Check sheet for the modelled part. Datum: model origin and axes. Units: mm. A direction names the side the tool comes from. Round coordinates to 2 decimals unless told otherwise and drop trailing zeros. Loops run counter-clockwise (first coordinate to the right, second up) from the corner with the lowest first, then second, coordinate; pieces in that order, holes last. Notation, with made-up numbers: (-28, 63.5) - (-13, 63.5) arc R11 cw to (-13, 72.5) - close; hole circle Ø4 at (60, 62). An arc over 180 degrees is marked (long way). Put each result on its own line as item: value.
```python
from build123d import *

# Parameters (mm, degrees)
SKETCH_R        = 31.9
SKETCH_R_2      = 6
PAD_DEPTH       = 2
SKETCH001_R     = 31.9
SKETCH001_R_2   = 30
PAD001_DEPTH    = 2
PAD002_DEPTH    = 2
CHAMFER_SIZE    = 1.9
CHAMFER001_SIZE = 0.3


with BuildPart() as part:
    # Sketch → Pad (new body)
    with BuildSketch(Plane.XY):
        Circle(SKETCH_R)
        with Locations((9.999037, 20.71278)):
            Circle(SKETCH_R_2, mode=Mode.SUBTRACT)
        with Locations((22.937312, 1.69697)):
            Circle(SKETCH_R_2, mode=Mode.SUBTRACT)
        with Locations((12.938275, -19.01581)):
            Circle(SKETCH_R_2, mode=Mode.SUBTRACT)
        with Locations((-9.999037, -20.71278)):
            Circle(SKETCH_R_2, mode=Mode.SUBTRACT)
        with Locations((-22.937312, -1.69697)):
            Circle(SKETCH_R_2, mode=Mode.SUBTRACT)
        with Locations((-12.938275, 19.01581)):
            Circle(SKETCH_R_2, mode=Mode.SUBTRACT)
        Polygon((0, 16.858628), (-14.6, 8.429314), (-14.6, -8.429314), (0, -16.858628), (14.6, -8.429314), (14.6, 8.429314), align=None, mode=Mode.SUBTRACT)
    extrude(amount=PAD_DEPTH)

    # Sketch001 (on Face15 of Pad) → Pad001 (join)
    with BuildSketch(Plane.XY.offset(2)):
        Circle(SKETCH001_R)
        Circle(SKETCH001_R_2, mode=Mode.SUBTRACT)
    extrude(amount=PAD001_DEPTH)

    # Sketch002 (on Face17 of Pad001) → Pad002 (join)
    with BuildSketch(Plane.XY.offset(2)):
        Polygon((0, 19.052559), (-16.5, 9.526279), (-16.5, -9.526279), (0, -19.052559), (16.5, -9.526279), (16.5, 9.526279), align=None)
        Polygon((0, 16.858628), (-14.6, 8.429314), (-14.6, -8.429314), (0, -16.858628), (14.6, -8.429314), (14.6, 8.429314), align=None, mode=Mode.SUBTRACT)
    extrude(amount=PAD002_DEPTH)

    # Chamfer
    chamfer_edges = [part.edges().sort_by_distance(p)[0] for p in [
        (-31.9, 0, 0),
    ]]
    chamfer(chamfer_edges, length=CHAMFER_SIZE)

    # Chamfer001
    chamfer001_edges = [part.edges().sort_by_distance(p)[0] for p in [
        (-7.3, -12.643971, 4),
        (-14.6, 0, 4),
        (-7.3, 12.643971, 4),
        (7.3, 12.643971, 4),
        (14.6, 0, 4),
        (7.3, -12.643971, 4),
    ]]
    chamfer(chamfer001_edges, length=CHAMFER001_SIZE)


solid = part.part
```
Item 1: Go/stop test with flat-tipped pins: pin 1 (1.5 mm diameter, centred on x = -25, z = 1, fed in from +Y); pin 2 (1 mm diameter, centred on x = 2, y = 25.5, fed in from +Z); pin 3 (2 mm diameter, centred on y = -20.5, z = 2, fed in from -X). Record where each tip stops, or that it passes through.
Filled sheet:
pin 1: y = 19.9
pin 2: z = 2
pin 3: x = -25.25
Item 2: Release check for a two-part mould opening along X. For faces 1 (the flat face through (14.6, 0, 2)), 2 (the flat face through (6, -14, 4)), 3 (the flat face through (-8.37, -14.22, 2.99)) record: +X half, -X half, draft (parallel to the pull), parting line (faces both ways), or undercut.
Filled sheet:
face 1: undercut
face 2: draft
face 3: undercut
Item 3: Section check A-A on z = 2.85. Enter the section's corners in (x, y), then the cut area to 3 significant figures.
Filled sheet:
outline: circle Ø63.8 at (0, 0); (-16.5, -9.53) - (0, -19.05) - (16.5, -9.53) - (16.5, 9.53) - (0, 19.05) - (-16.5, 9.53) - close; hole circle Ø60 at (0, 0); hole (-14.6, -8.43) - (0, -16.86) - (14.6, -8.43) - (14.6, 8.43) - (0, 16.86) - (-14.6, 8.43) - close
area: 574 mm²
Item 4: Section check C-C on x = 8.5. Count the separate pieces of the cut face and the enclosed holes in it, then the cut area to 3 significant figures.
Filled sheet:
separate pieces: 4
enclosed holes: 0
area: 48.6 mm²
Item 5: Tool access check on faces 4 (the flat face through (-7.2, 12.7, 1.8)), 5 (the flat face through (8.37, 14.22, 2.99)). Record the directions out of +Z, -Z, +X, -X, +Y, -Y that give a thin tool (end or side, any length) a straight path to the whole face; none if there is none.
Filled sheet:
face 4: +Z, -Z
face 5: +Z
Item 6: Thickness scan on line 1 (X direction, y = -21.5, z = 1.8); line 2 (X direction, y = 19, z = 3); line 3 (X direction, y = 8, z = 3.75). Record the ranges inside material, lowest first. Write a range as from..to.
Filled sheet:
line 1: -23.43..-15.95, -4.05..7.48, 18.4..23.43
line 2: -25.62..-23.22, -0.09..0.09, 23.22..25.62
line 3: -30.88..-28.91, -16.5..-14.65, 14.65..16.5, 28.91..30.88
Item 7: Section check B-B on y = 0. Enter the section's corners in (x, z), then the cut area to 3 significant figures.
Filled sheet:
outline: (-31.9, 1.9) - (-30, 0) - (-28.69, 0) - (-28.69, 2) - (-30, 2) - (-30, 4) - (-31.9, 4) - close; (-17.18, 0) - (-14.6, 0) - (-14.6, 3.7) - (-14.9, 4) - (-16.5, 4) - (-16.5, 2) - (-17.18, 2) - close; (14.6, 0) - (17.18, 0) - (17.18, 2) - (16.5, 2) - (16.5, 4) - (14.9, 4) - (14.6, 3.7) - close; (28.69, 0) - (30, 0) - (31.9, 1.9) - (31.9, 4) - (30, 4) - (30, 2) - (28.69, 2) - close
area: 34.7 mm²
